from build123d import *

# Parameters (mm, degrees)
SKETCH_1_R          = 14.4
SKETCH_1_R_2        = 9
EXTRUDE_1_DEPTH     = 3
SKETCH_2_R          = 9.75
CUT_EXTRUDE_1_DEPTH = 0.8
SKETCH_3_R          = 0.8
CUT_EXTRUDE_2_DEPTH = 10
SKETCH_4_R          = 4
CUT_EXTRUDE_3_DEPTH = 10
FILLET_1_R          = 1


with BuildPart() as part:
    # 草图1 → 凸台-拉伸1 (new body)
    with BuildSketch(Plane.XY):
        Circle(SKETCH_1_R)
        Circle(SKETCH_1_R_2, mode=Mode.SUBTRACT)
    extrude(amount=EXTRUDE_1_DEPTH)

    # 草图2 → 切除-拉伸1 (cut)
    with BuildSketch(Plane.XY.offset(3)):
        Circle(SKETCH_2_R)
    extrude(amount=-CUT_EXTRUDE_1_DEPTH, mode=Mode.SUBTRACT)

    # 草图3 → 切除-拉伸2 (cut)
    with BuildSketch(Plane.XY.offset(3)):
        with Locations((0, 13)):
            Circle(SKETCH_3_R)
        with Locations((11.258330249, 6.5)):
            Circle(SKETCH_3_R)
        with Locations((11.258330249, -6.5)):
            Circle(SKETCH_3_R)
        with Locations((0, -13)):
            Circle(SKETCH_3_R)
        with Locations((-11.258330249, -6.5)):
            Circle(SKETCH_3_R)
        with Locations((-11.258330249, 6.5)):
            Circle(SKETCH_3_R)
    extrude(amount=-CUT_EXTRUDE_2_DEPTH, mode=Mode.SUBTRACT)

    # 草图4 → 切除-拉伸3 (cut)
    with BuildSketch(Plane.XY.offset(3)):
        with Locations((7.267001819, 12.431841559)):
            Circle(SKETCH_4_R)
        with Locations((14.399791516, -0.077487405)):
            Circle(SKETCH_4_R)
        with Locations((7.132789697, -12.509328965)):
            Circle(SKETCH_4_R)
        with Locations((-7.267001819, -12.431841559)):
            Circle(SKETCH_4_R)
        with Locations((-14.399791516, 0.077487405)):
            Circle(SKETCH_4_R)
        with Locations((-7.132789697, 12.509328965)):
            Circle(SKETCH_4_R)
    extrude(amount=-CUT_EXTRUDE_3_DEPTH, mode=Mode.SUBTRACT)

    # 圆角1
    fillet_1_edges = [part.edges().sort_by_distance(p)[0] for p in [
        (3.566819155, 13.951265216, 1.5),
        (10.406459035, 9.953170869, 1.5),
        (13.865559669, 3.886676609, 1.5),
        (13.822928338, -4.035672453, 1.5),
        (10.298740514, -10.064588606, 1.5),
        (3.416469303, -13.988843322, 1.5),
        (-3.566819155, -13.951265216, 1.5),
        (-10.406459035, -9.953170869, 1.5),
        (-13.865559669, -3.886676609, 1.5),
        (-13.822928338, 4.035672453, 1.5),
        (-10.298740514, 10.064588606, 1.5),
        (-3.416469303, 13.988843322, 1.5),
    ]]
    fillet(fillet_1_edges, radius=FILLET_1_R)


solid = part.part
CAD build for the part. Positions are in the model's coordinates, mm. A direction names the side the tool comes from. Coordinates: 2 decimals unless noted, no trailing zeros. Loops run counter-clockwise (first coordinate to the right, second up) from the corner with the lowest first, then second, coordinate; pieces in that order, holes last. Notation, with made-up numbers: (65.5, 5) - (83.5, 5) arc R30 ccw to (83.5, 28) - close; hole circle Ø7 at (-3.5, -9.5). An arc over 180 degrees is marked (long way). Use one line per item in the form item = value. Start each with the question number.
1) Band-saw the part on D-D (x = 8.5). Give the cut face in (y, z), and give its area (3 significant figures).
2) Two-plate mould, pull along Y, no slides. Class faces 1 (the face through (12.53, 7.1, 1.48)), 2 (the face through (-10.4, 0, 1.5)), 3 (the face through (-0.1, -14.4, 1.5)): +Y half, -Y half, draft (parallel to the pull), parting line (faces both ways), or undercut.
3) Band-saw the part on B-B (y = -0.5). Give the cut face in (x, z), and give its area (3 significant figures).
4) Flat gauge pins, fed straight in: pin 1 (1.4 mm diameter, centred on x = 11.26, y = 6.5, fed in from -Z); pin 2 (1 mm diameter, centred on y = 11, z = 2, fed in from +X). Where does each tip first touch, or does it go through?
5) Drill centre lines: L1, parallel to Y at x = 0, z = 1.7; L2, parallel to Y at x = -11.5, z = 2.65; L3, parallel to Y at x = 10.25, z = 1.95. Where is each one in solid material? Low to high. Write a range as from..to.
6) Band-saw the part on C-C (y = 6.5). Give the cut face in (x, z), and give its area (3 significant figures).
7) Band-saw the part on A-A (x = 0). Give the cut face in (y, z), and give its area (3 significant figures).
8) Tool access for faces 4 (the face through (12.415, -7.296, 1.479)), 5 (the face through (3, -9, 2.2)): list every direction of +Z, -Z, +X, -X, +Y, -Y with a clear straight run to the whole face (end or side of a thin tool).
Check values:
q1.outline = (-8.75, 0) - (-2.96, 0) - (-2.96, 2.2) - (-4.78, 2.2) - (-4.78, 3) - (-8.75, 3) - close; (2.96, 0) - (8.63, 0) - (8.63, 3) - (4.78, 3) - (4.78, 2.2) - (2.96, 2.2) - close
q1.area = 31.5 mm2
q2.face_1 = +Y half
q2.face_2 = undercut
q2.face_3 = -Y half
q3.outline = (-10.44, 0) - (-8.99, 0) - (-8.99, 2.2) - (-9.74, 2.2) - (-9.74, 3) - (-10.44, 3) - close; (8.99, 0) - (10.42, 0) - (10.42, 3) - (9.74, 3) - (9.74, 2.2) - (8.99, 2.2) - close
q3.area = 7.47 mm2
q4.pin_1 = through
q4.pin_2 = 3.76
q5.L1 = -14.4..-13.8, -12.2..-9, 9..12.2, 13.8..14.4
q5.L2 = -8.67..-7.26, -5.74..-2.68, 2.83..5.74, 7.26..8.67
q5.L3 = -9.61..9.5
q6.outline = (-12.85, 0) - (-12.06, 0) - (-12.06, 3) - (-12.85, 3) - close; (-10.46, 0) - (-6.22, 0) - (-6.22, 2.2) - (-7.27, 2.2) - (-7.27, 3) - (-10.46, 3) - close; (6.22, 0) - (10.46, 0) - (10.46, 3) - (7.27, 3) - (7.27, 2.2) - (6.22, 2.2) - close; (12.06, 0) - (12.85, 0) - (12.85, 3) - (12.06, 3) - close
q6.area = 28.5 mm2
q7.outline = (-14.4, 0) - (-13.8, 0) - (-13.8, 3) - (-14.4, 3) - close; (-12.2, 0) - (-9, 0) - (-9, 2.2) - (-9.75, 2.2) - (-9.75, 3) - (-12.2, 3) - close; (9, 0) - (12.2, 0) - (12.2, 3) - (9.75, 3) - (9.75, 2.2) - (9, 2.2) - close; (13.8, 0) - (14.4, 0) - (14.4, 3) - (13.8, 3) - close
q7.area = 21.6 mm2
q8.face_4 = +Z, -Z, +X, -Y
q8.face_5 = +Z
